```python
from build123d import *

# Parameters (mm, degrees)
SKETCH1_W                               = 50
SKETCH1_H                               = 30
BOSS_EXTRUDE1_DEPTH                     = 60
SKETCH2_R                               = 6
BOSS_EXTRUDE2_DEPTH                     = 22
SKETCH3_W                               = 16
SKETCH3_H                               = 12
CUT_EXTRUDE1_DEPTH                      = 99.488578018
SKETCH4_W                               = 22
SKETCH4_H                               = 12
CUT_EXTRUDE2_DEPTH                      = 99.488578018
CUT_EXTRUDE3_REACH                      = 100.489
CBORE_FOR_M6_HEX_HEAD_BOLT2_D           = 6.6
CBORE_FOR_M6_HEX_HEAD_BOLT2_CBORE_D     = 14.547
CBORE_FOR_M6_HEX_HEAD_BOLT2_CBORE_DEPTH = 4


with BuildPart() as part:
    # Sketch1 → Boss-Extrude1 (new body)
    with BuildSketch(Plane.XY):
        with Locations((25, 15)):
            Rectangle(SKETCH1_W, SKETCH1_H)
    extrude(amount=-BOSS_EXTRUDE1_DEPTH)

    # Sketch2 → Boss-Extrude2 (add)
    with BuildSketch(Plane(origin=(0, 0, -60), x_dir=(-1, 0, 0), z_dir=(0, 0, -1))):
        with BuildLine():
            Line((-50, 30), (-33.373426859, 55.466783574))
            ThreePointArc((-33.373426859, 55.466783574), (-25, 60), (-16.626573141, 55.466783574))
            Line((-16.626573141, 55.466783574), (0, 30))
            Line((0, 30), (-50, 30))
        make_face()
        with Locations((-25, 50)):
            Circle(SKETCH2_R, mode=Mode.SUBTRACT)
    extrude(amount=-BOSS_EXTRUDE2_DEPTH)

    # Sketch3 → Cut-Extrude1 (cut, through all)
    with BuildSketch(Plane(origin=(50, 0, 0), x_dir=(0, 0, -1), z_dir=(1, 0, 0))):
        with Locations((30, 24)):
            Rectangle(SKETCH3_W, SKETCH3_H)
    extrude(amount=-CUT_EXTRUDE1_DEPTH, mode=Mode.SUBTRACT)

    # Sketch4 → Cut-Extrude2 (cut, through all)
    with BuildSketch(Plane.XY):
        with Locations((25, 6)):
            Rectangle(SKETCH4_W, SKETCH4_H)
    extrude(amount=-CUT_EXTRUDE2_DEPTH, mode=Mode.SUBTRACT)

    # Sketch5 → Cut-Extrude3 (cut, up to next)
    with BuildSketch(Plane.XY, mode=Mode.PRIVATE) as cut_extrude3_sk1:
        Polygon((50, 30), (50, 23), (43, 30), align=None)
    cut_extrude3_tool1 = extrude(cut_extrude3_sk1.sketch, amount=-CUT_EXTRUDE3_REACH, mode=Mode.PRIVATE) & part.part
    # Sketch5 → Cut-Extrude3 (cut, up to next)
    with BuildSketch(Plane.XY, mode=Mode.PRIVATE) as cut_extrude3_sk2:
        Polygon((0, 23), (0, 30), (7, 30), align=None)
    cut_extrude3_tool2 = extrude(cut_extrude3_sk2.sketch, amount=-CUT_EXTRUDE3_REACH, mode=Mode.PRIVATE) & part.part
    add(cut_extrude3_tool1.solids().sort_by_distance((47.666667, 27.666667, 0))[0], mode=Mode.SUBTRACT)
    add(cut_extrude3_tool2.solids().sort_by_distance((2.333333, 27.666667, 0))[0], mode=Mode.SUBTRACT)

    # CBORE for M6 Hex Head Bolt2 (through all)
    with Locations(Plane(origin=(0, 30, 0), x_dir=(1, 0, 0), z_dir=(0, 1, 0))):
        with Locations((25, 11)):
            CounterBoreHole(CBORE_FOR_M6_HEX_HEAD_BOLT2_D / 2, CBORE_FOR_M6_HEX_HEAD_BOLT2_CBORE_D / 2, CBORE_FOR_M6_HEX_HEAD_BOLT2_CBORE_DEPTH)


solid = part.part
```
The listing builds one solid part. Answer for the finished solid, in the listing's coordinates (mm). A direction names the side the tool comes from. Coordinates: 2 decimals unless noted, no trailing zeros. Write each loop counter-clockwise with the first axis right and the second up, starting at its lowest first coordinate (ties: lowest second). Pieces come first, ordered by that corner, then holes. Notation, with made-up numbers: (-24, 18) - (-12, 18) arc R22 ccw to (-12, 28) - close; hole circle Ø8 at (79.5, -35). An arc over 180 degrees is marked (long way). Return JSON: item names as keys, results as strings. Group by question number.
1. A cutting plane is placed at C-C, the plane x = 25. Determine the outline of the cut face in (y, z), plus the area to 3 significant figures.
2. Straight lines are drawn through the part: L1, parallel to Z at x = 25, y = 22; L2, parallel to Y at x = 25, z = -47.5; L3, parallel to X at y = 8, z = -6.5. For each, find the intervals that lie inside material, in ascending order.
3. Given pin 1 (5 mm diameter, centred on x = 35.5, z = -30.5, fed in from +Y); pin 2 (4 mm diameter, centred on y = 30, z = -21, fed in from -X); pin 3 (5 mm diameter, centred on x = 16.5, y = 50.5, fed in from +Z); pin 4 (12.5 mm diameter, centred on x = 19, y = 30.5, fed in from +Z), each flat-ended and moving along its own axis, determine where each tip first touches the part or whether it passes through.
4. Which of the six approach directions +Z, -Z, +X, -X, +Y, -Y give full straight-line access (tool end or side, diameter ignored) to faces 1 (the flat face through (4, 27, -11)), 2 (the flat face through (25, 35, -38)), 3 (the flat face through (14, 6, -30))?
5. A cutting plane is placed at A-A, the plane y = 11. Determine the outline of the cut face in (x, z).
6. A cutting plane is placed at D-D, the plane z = -29.5. Determine the outline of the cut face in (x, y), plus the area to 3 significant figures.
7. Determine the mould class of faces 4 (the flat face through (43, 0, -30)), 5 (the flat face through (25, 24, -22)), 6 (the flat face through (25, 18, -30)), 7 (the flat face through (25, 19, 0)) for opening direction Z: released by +Z, released by -Z, zero draft, split by the parting line, or undercut.
8. A cutting plane is placed at B-B, the plane z = -11. Determine the outline of the cut face in (x, y).
Ans:
{
 "1": {"outline": "(12, -60) - (44, -60) - (44, -38) - (18, -38) - (18, -22) - (30, -22) - (30, -18.27) - (26, -18.27) - (26, -14.3) - (12, -14.3) - close; (12, -7.7) - (26, -7.7) - (26, -3.73) - (30, -3.73) - (30, 0) - (12, 0) - close; (56, -60) - (60, -60) - (60, -38) - (56, -38) - close", "area": "1,130 mm²"},
 "2": {"L1": "-60 to -38, -22 to -14.3, -7.7 to 0", "L2": "12 to 44, 56 to 60", "L3": "0 to 14, 36 to 50"},
 "3": {"pin 1": "y = 18", "pin 2": "x = 5", "pin 3": "z = -38", "pin 4": "z = 0"},
 "4": {"face 1": "+Z, -X, +Y", "face 2": "+X, -X, +Y", "face 3": "+Z, -Z, -Y"},
 "5": {"outline": "(0, -60) - (14, -60) - (14, 0) - (0, 0) - close; (36, -60) - (50, -60) - (50, 0) - (36, 0) - close"},
 "6": {"outline": "(0, 0) - (14, 0) - (14, 12) - (36, 12) - (36, 0) - (50, 0) - (50, 18) - (0, 18) - close", "area": "636 mm²"},
 "7": {"face 4": "zero draft", "face 5": "undercut", "face 6": "undercut", "face 7": "released by +Z"},
 "8": {"outline": "(0, 0) - (14, 0) - (14, 12) - (21.7, 12) - (21.7, 26) - (17.73, 26) - (17.73, 30) - (7, 30) - (0, 23) - close; (28.3, 12) - (36, 12) - (36, 0) - (50, 0) - (50, 23) - (43, 30) - (32.27, 30) - (32.27, 26) - (28.3, 26) - close"}
}
